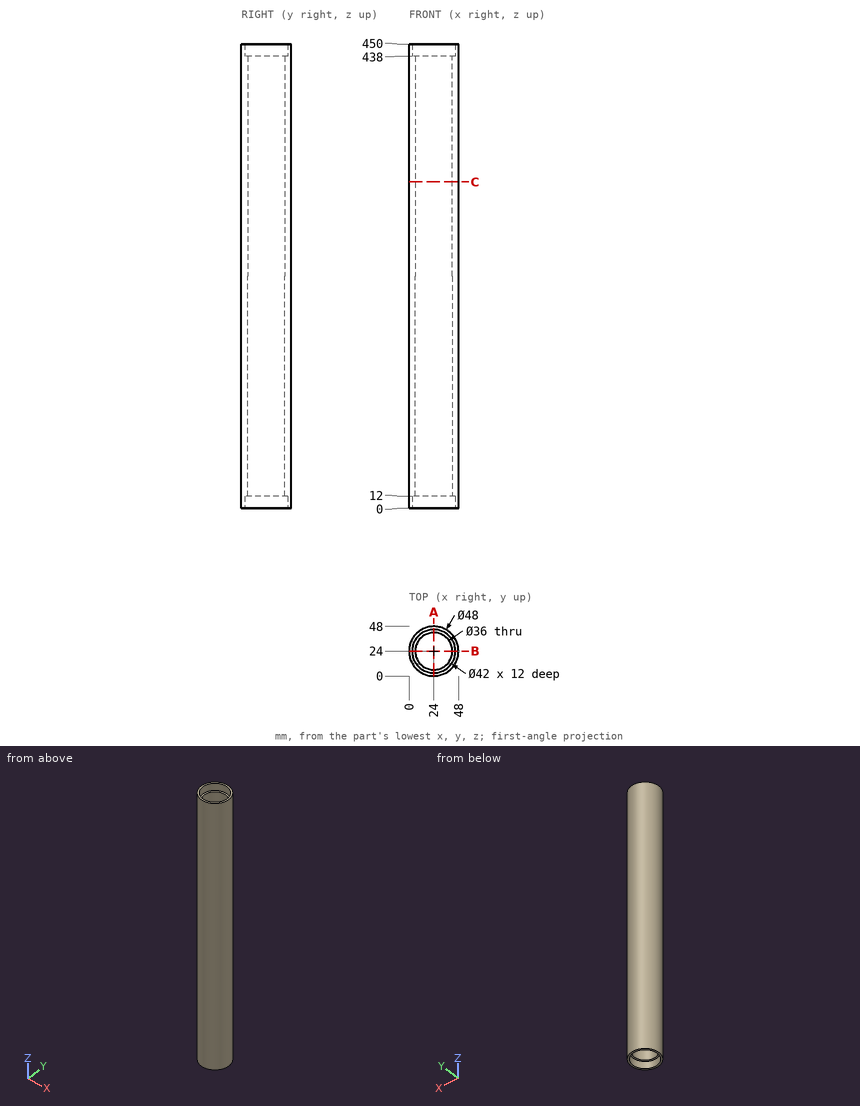
Check sheet for the drawn part. Datum: minimum x, y, z corner. Units: mm. Round coordinates to 2 decimals unless told otherwise and drop trailing zeros. Order: outer loops, then holes, each group sorted by start corner. A loop starts at its lowest first (then second) coordinate and runs counter-clockwise, first axis right, second up. Notation, with made-up numbers: (10, 64) - (16, 64) arc R26 ccw to (16, 89) - close; hole circle Ø7 at (46, 6.5). An arc over 180 degrees is marked (long way). Use a Markdown table: item, result. Add a question column.
(1) Sectioned sample at C-C, the plane z = 316.5. Enter the section's corners in (x, y), and give its area (3 significant figures).
(2) Material ranges on line 1 along Y through (x, z) = (24, 443.5); line 2 along X through (y, z) = (14, 227.5); line 3 along X through (y, z) = (21, 195.5), recorded low to high. Write a range as [from, to].
(3) Sectioned sample at A-A, the plane x = 24. Enter the section's corners in (y, z).
(4) Depth check by flat-ended pin: pin 1 (4 mm diameter, centred on y = 27, z = 221.5, fed in from +X); pin 2 (1 mm diameter, centred on x = 16.5, y = 8, fed in from -Z); pin 3 (8 mm diameter, centred on y = 8.5, z = 384, fed in from -X); pin 4 (21 mm diameter, centred on x = 16, y = 16.5, fed in from +Z). Enter the tip coordinate at first touch or a pass-through.
Answers below:
| question | item | result |
|---|---|---|
| 1 | outline | circle Ø48 at (24, 24); hole circle Ø36 at (24, 24) |
| 1 | area | 792 mm² |
| 2 | line 1 | [0, 3], [45, 48] |
| 2 | line 2 | [2.18, 9.03], [38.97, 45.82] |
| 2 | line 3 | [0.19, 6.25], [41.75, 47.81] |
| 3 | outline | (0, 0) - (3, 0) - (3, 12) - (6, 12) - (6, 438) - (3, 438) - (3, 450) - (0, 450) - close; (42, 12) - (45, 12) - (45, 0) - (48, 0) - (48, 450) - (45, 450) - (45, 438) - (42, 438) - close |
| 4 | pin 1 | x = 47.98 |
| 4 | pin 2 | z = 12 |
| 4 | pin 3 | x = 2.93 |
| 4 | pin 4 | z = 450 |
